Here's how the part is built. I have some questions about the finished solid (model axes, mm). A direction names the side the tool comes from. Round coordinates to 2 decimals unless told otherwise and drop trailing zeros. Order: outer loops, then holes, each group sorted by start corner. A loop starts at its lowest first (then second) coordinate and runs counter-clockwise, first axis right, second up. Notation, with made-up numbers: (62, 82) - (108, 82) arc R15 ccw to (108, 104) - close; hole circle Ø11 at (58, 71.25). An arc over 180 degrees is marked (long way). One line per item, written item: value.
from build123d import *

# Parameters (mm, degrees)
CROQUIS2_R                 = 1.6
SALIENTE_EXTRUIR1_DEPTH    = 15.1
CORTAR_EXTRUIR4_DEPTH      = 8.1
CORTAR_EXTRUIR2_DEPTH      = 37.049965326
CORTAR_EXTRUIR2_DEPTH_BACK = 4
CROQUIS4_R                 = 3.25
CORTAR_EXTRUIR3_DEPTH      = 4
REDONDEO2_R                = 1
CHAFL_N1_SIZE              = 0.5


with BuildPart() as part:
    # Croquis2 → Saliente-Extruir1 (new, symmetric)
    with BuildSketch(Plane(origin=(0, 0, 0), x_dir=(0, 0, -1), z_dir=(0, 1, 0))):
        with BuildLine():
            Line((0, -7), (0, 7))
            Line((0, 7), (-9, 7))
            Line((-9, 7), (-9, 5.817215829))
            ThreePointArc((-9, 5.817215829), (-9.710647783, 4.541706881), (-11.169230769, 4.474781407))
            ThreePointArc((-11.169230769, 4.474781407), (-18.4, 0), (-11.169230769, -4.474781407))
            ThreePointArc((-11.169230769, -4.474781407), (-9.710647783, -4.541706881), (-9, -5.817215829))
            Line((-9, -5.817215829), (-9, -7))
            Line((-9, -7), (0, -7))
        make_face()
        with Locations(Location((-13.4, 0, 0), (0, 0, 180))):
            Circle(CROQUIS2_R, mode=Mode.SUBTRACT)
    extrude(amount=SALIENTE_EXTRUIR1_DEPTH, both=True)

    # Croquis6 → Cortar-Extruir4 (cut, symmetric)
    with BuildSketch(Plane(origin=(0, 0, 0), x_dir=(1, 0, 0), z_dir=(0, 1, 0))):
        with BuildLine():
            Line((-7, -9), (-3.3, -9))
            ThreePointArc((-3.3, -9), (0, -7.9), (3.3, -9))
            Line((3.3, -9), (7, -9))
            Line((7, -9), (7, -18.9))
            Line((7, -18.9), (-7, -18.9))
            Line((-7, -18.9), (-7, -9))
        make_face()
    extrude(amount=CORTAR_EXTRUIR4_DEPTH, both=True, mode=Mode.SUBTRACT)

    # Croquis4 → Cortar-Extruir2 (cut, two sides: drawn at the far end of the back side and taken through both)
    with BuildSketch(Plane(origin=(0, 15.1, 0), x_dir=(1, 0, 0), z_dir=(0, 1, 0)).offset(-CORTAR_EXTRUIR2_DEPTH_BACK)):
        with Locations(Location((0, -13.4, 0), (0, 0, 90))):
            Circle(CROQUIS4_R)
    extrude(amount=CORTAR_EXTRUIR2_DEPTH + CORTAR_EXTRUIR2_DEPTH_BACK, mode=Mode.SUBTRACT)

    # Croquis5 → Cortar-Extruir3 (cut)
    with BuildSketch(Plane.XZ.offset(15.1)):
        Polygon((1.5011107, 10.8), (3.0022214, 13.4), (1.5011107, 16), (-1.5011107, 16), (-3.0022214, 13.4), (-1.5011107, 10.8), align=None)
    extrude(amount=-CORTAR_EXTRUIR3_DEPTH, mode=Mode.SUBTRACT)

    # Redondeo2
    redondeo2_edges = [part.edges().sort_by_distance(p)[0] for p in [
        (7, 0, 9),
        (-7, 0, 9),
    ]]
    fillet(redondeo2_edges, radius=REDONDEO2_R)

    # Chaflán1
    # the kernel refuses this chamfer: 0.5 mm, written as the material it takes off along each edge
    with BuildSketch(Plane(origin=(0, -15.1, 13.4), x_dir=(-0.8949562813691682, 0, -0.44615384615384657), z_dir=(0.44615384615384657, 0, -0.8949562813691682))) as chafl_n1_piece_1:
        Polygon((5 - CHAFL_N1_SIZE, 0), (5, CHAFL_N1_SIZE), (5, 0), align=None)
    revolve(axis=Axis((0, -15.1, 13.4), (0, 1, 0)), revolution_arc=232.994370335, mode=Mode.SUBTRACT)
    with BuildSketch(Plane(origin=(-5.817215829, -15.1, 10.5), x_dir=(0, 0, -1), z_dir=(-1, 0, 0))) as chafl_n1_piece_2:
        Polygon((1.5 + CHAFL_N1_SIZE, 0), (1.5, -CHAFL_N1_SIZE), (1.5, 0), align=None)
    revolve(axis=Axis((-5.817215829, -15.1, 10.5), (0, -1, 0)), revolution_arc=116.497185168, mode=Mode.SUBTRACT)
    with BuildSketch(Plane(origin=(-7, -15.1, -1.285841494), x_dir=(0.9996219169112968, -0.027495876610585647, 0), z_dir=(0, 0, 1)), Plane(origin=(-7, 15.1, -1.285841494), x_dir=(-0.027495876610585647, -0.9996219169112968, 0), z_dir=(0, 0, 1)), Plane(origin=(7, -15.1, 8), x_dir=(-0.9996219169112968, -0.027495876610585647, 0), z_dir=(0, 0, -1)), Plane(origin=(7, 15.1, 8), x_dir=(0.027495876610585647, -0.9996219169112968, 0), z_dir=(0, 0, -1))) as chafl_n1_piece_3:
        Polygon((CHAFL_N1_SIZE * 0.999621916911, CHAFL_N1_SIZE * 0.0274958766106), (-CHAFL_N1_SIZE * 0.0274958766106, CHAFL_N1_SIZE * 0.999621916911), (0, 0), align=None)
    extrude(amount=9.285841494, mode=Mode.SUBTRACT)
    with BuildSketch(Plane(origin=(-5.817215829, 15.1, 10.5), x_dir=(0, 0, -1), z_dir=(-1, 0, 0))) as chafl_n1_piece_4:
        Polygon((1.5 + CHAFL_N1_SIZE, 0), (1.5, CHAFL_N1_SIZE), (1.5, 0), align=None)
    revolve(axis=Axis((-5.817215829, 15.1, 10.5), (0, -1, 0)), revolution_arc=116.497185168, mode=Mode.SUBTRACT)
    with BuildSketch(Plane(origin=(0, 15.1, 13.4), x_dir=(-0.8949562813691682, 0, -0.44615384615384657), z_dir=(0.44615384615384657, 0, -0.8949562813691682))) as chafl_n1_piece_5:
        Polygon((5 - CHAFL_N1_SIZE, 0), (5, -CHAFL_N1_SIZE), (5, 0), align=None)
    revolve(axis=Axis((0, 15.1, 13.4), (0, 1, 0)), revolution_arc=232.994370335, mode=Mode.SUBTRACT)
    with BuildSketch(Plane(origin=(5.817215829, 15.1, 10.5), x_dir=(-0.8949562813691686, 0, 0.44615384615384585), z_dir=(0.44615384615384585, 0, 0.8949562813691686))) as chafl_n1_piece_6:
        Polygon((1.5 + CHAFL_N1_SIZE, 0), (1.5, CHAFL_N1_SIZE), (1.5, 0), align=None)
    revolve(axis=Axis((5.817215829, 15.1, 10.5), (0, -1, 0)), revolution_arc=116.497185168, mode=Mode.SUBTRACT)
    with BuildSketch(Plane(origin=(5.817215829, 15.1, 9), x_dir=(0, -0.9996219169112968, 0.027495876610585647), z_dir=(1, 0, 0)), Plane(origin=(-6, -15.1, 9), x_dir=(0, -0.027495876610585647, -0.9996219169112968), z_dir=(1, 0, 0)), Plane(origin=(-6, 15.1, 9), x_dir=(0, -0.9996219169112968, 0.027495876610585647), z_dir=(1, 0, 0)), Plane(origin=(5.817215829, -15.1, 9), x_dir=(0, -0.027495876610585647, -0.9996219169112968), z_dir=(1, 0, 0))) as chafl_n1_piece_7:
        Polygon((CHAFL_N1_SIZE * 0.999621916911, CHAFL_N1_SIZE * 0.0274958766106), (-CHAFL_N1_SIZE * 0.0274958766106, CHAFL_N1_SIZE * 0.999621916911), (0, 0), align=None)
    extrude(amount=0.182784171, mode=Mode.SUBTRACT)
    with BuildSketch(Plane(origin=(-5.817215829, 8.1, 10.5), x_dir=(0.8949562813691686, 0, 0.44615384615384585), z_dir=(-0.44615384615384585, 0, 0.8949562813691686))) as chafl_n1_piece_8_section:
        Polygon((1.5 + CHAFL_N1_SIZE, 0), (1.5, CHAFL_N1_SIZE), (1.5, 0), align=None)
    chafl_n1_piece_8 = revolve(axis=Axis((-5.817215829, 8.1, 10.5), (0, 1, 0)), revolution_arc=165.645776503, mode=Mode.PRIVATE)
    chafl_n1_piece_8 = split(chafl_n1_piece_8, bisect_by=Plane(origin=(-4.168851262, 8.241008039, 9), z_dir=(0, 0, 1)), keep=Keep.TOP, mode=Mode.PRIVATE)
    add(chafl_n1_piece_8, mode=Mode.SUBTRACT)
    with BuildSketch(Plane(origin=(0, 8.1, 13.4), x_dir=(-0.8949562813691682, 0, -0.44615384615384657), z_dir=(0.44615384615384657, 0, -0.8949562813691682))) as chafl_n1_piece_9:
        Polygon((5 - CHAFL_N1_SIZE, 0), (5, CHAFL_N1_SIZE), (5, 0), align=None)
    revolve(axis=Axis((0, 8.1, 13.4), (0, 1, 0)), revolution_arc=232.994370335, mode=Mode.SUBTRACT)
    with BuildSketch(Plane(origin=(5.817215829, 8.1, 10.5), x_dir=(0.7564084690774899, 0, -0.6540995550433039), z_dir=(0.6540995550433039, 0, 0.7564084690774899))) as chafl_n1_piece_10_section:
        Polygon((1.5, CHAFL_N1_SIZE), (1.5 + CHAFL_N1_SIZE, 0), (1.5, 0), align=None)
    chafl_n1_piece_10 = revolve(axis=Axis((5.817215829, 8.1, 10.5), (0, 1, 0)), revolution_arc=165.645776503, mode=Mode.PRIVATE)
    chafl_n1_piece_10 = split(chafl_n1_piece_10, bisect_by=Plane(origin=(4.495767194, 8.276282953, 9), z_dir=(0, 0, 1)), keep=Keep.TOP, mode=Mode.PRIVATE)
    add(chafl_n1_piece_10, mode=Mode.SUBTRACT)
    with BuildSketch(Plane(origin=(-5.817215829, -8.1, 10.5), x_dir=(0.8949562813691686, 0, 0.44615384615384585), z_dir=(-0.44615384615384585, 0, 0.8949562813691686))) as chafl_n1_piece_11_section:
        Polygon((1.5, -CHAFL_N1_SIZE), (1.5 + CHAFL_N1_SIZE, 0), (1.5, 0), align=None)
    chafl_n1_piece_11 = revolve(axis=Axis((-5.817215829, -8.1, 10.5), (0, 1, 0)), revolution_arc=165.645776503, mode=Mode.PRIVATE)
    chafl_n1_piece_11 = split(chafl_n1_piece_11, bisect_by=Plane(origin=(-4.495767364, -8.276282993, 9), z_dir=(0, 0, 1)), keep=Keep.TOP, mode=Mode.PRIVATE)
    add(chafl_n1_piece_11, mode=Mode.SUBTRACT)
    with BuildSketch(Plane(origin=(0, -8.1, 13.4), x_dir=(-0.8949562813691682, 0, -0.44615384615384657), z_dir=(0.44615384615384657, 0, -0.8949562813691682))) as chafl_n1_piece_12:
        Polygon((5, -CHAFL_N1_SIZE), (5 - CHAFL_N1_SIZE, 0), (5, 0), align=None)
    revolve(axis=Axis((0, -8.1, 13.4), (0, 1, 0)), revolution_arc=232.994370335, mode=Mode.SUBTRACT)
    with BuildSketch(Plane(origin=(5.817215829, -8.1, 10.5), x_dir=(0.7564084690774899, 0, -0.6540995550433039), z_dir=(0.6540995550433039, 0, 0.7564084690774899))) as chafl_n1_piece_13_section:
        Polygon((1.5, -CHAFL_N1_SIZE), (1.5 + CHAFL_N1_SIZE, 0), (1.5, 0), align=None)
    chafl_n1_piece_13 = revolve(axis=Axis((5.817215829, -8.1, 10.5), (0, 1, 0)), revolution_arc=165.645776503, mode=Mode.PRIVATE)
    chafl_n1_piece_13 = split(chafl_n1_piece_13, bisect_by=Plane(origin=(4.495767194, -8.276282953, 9), z_dir=(0, 0, 1)), keep=Keep.TOP, mode=Mode.PRIVATE)
    add(chafl_n1_piece_13, mode=Mode.SUBTRACT)
    with BuildSketch(Plane(origin=(6, -15.1, 8), x_dir=(1, 0, 0), z_dir=(0, 0, -1))) as chafl_n1_piece_14:
        Polygon((1 - CHAFL_N1_SIZE, 0), (1, -CHAFL_N1_SIZE), (1, 0), align=None)
    revolve(axis=Axis((6, -15.1, 8), (0, -1, 0)), revolution_arc=90, mode=Mode.SUBTRACT)
    with BuildSketch(Plane(origin=(-6, -15.1, 8), x_dir=(-1, 0, 0), z_dir=(0, 0, -1))) as chafl_n1_piece_15:
        Polygon((1 - CHAFL_N1_SIZE, 0), (1, CHAFL_N1_SIZE), (1, 0), align=None)
    revolve(axis=Axis((-6, -15.1, 8), (0, 1, 0)), revolution_arc=90, mode=Mode.SUBTRACT)
    with BuildSketch(Plane(origin=(6, 15.1, 8), x_dir=(1, 0, 0), z_dir=(0, 0, -1))) as chafl_n1_piece_16:
        Polygon((1, CHAFL_N1_SIZE), (1 - CHAFL_N1_SIZE, 0), (1, 0), align=None)
    revolve(axis=Axis((6, 15.1, 8), (0, -1, 0)), revolution_arc=90, mode=Mode.SUBTRACT)
    with BuildSketch(Plane(origin=(5.817215829, -15.1, 10.5), x_dir=(-0.8949562813691686, 0, 0.44615384615384585), z_dir=(0.44615384615384585, 0, 0.8949562813691686))) as chafl_n1_piece_17:
        Polygon((1.5 + CHAFL_N1_SIZE, 0), (1.5, -CHAFL_N1_SIZE), (1.5, 0), align=None)
    revolve(axis=Axis((5.817215829, -15.1, 10.5), (0, -1, 0)), revolution_arc=116.497185168, mode=Mode.SUBTRACT)
    with BuildSketch(Plane(origin=(-6, 15.1, 8), x_dir=(-1, 0, 0), z_dir=(0, 0, -1))) as chafl_n1_piece_18:
        Polygon((1, -CHAFL_N1_SIZE), (1 - CHAFL_N1_SIZE, 0), (1, 0), align=None)
    revolve(axis=Axis((-6, 15.1, 8), (0, 1, 0)), revolution_arc=90, mode=Mode.SUBTRACT)


solid = part.part
Q1. If we section it at C-C, the plane z = 13: Give the number of separate pieces and of enclosed holes in the cut face, then the cut area to 3 significant figures.
Results list:
separate pieces: 4
enclosed holes: 0
area: 72.0 mm²
Q2. If we section it at A-A, the plane x = 0: Please give me the cut outline in (y, z).
Results list:
outline: (-15.1, 0) - (15.1, 0) - (15.1, 10.15) - (11.1, 10.15) - (11.1, 11.8) - (8.1, 11.8) - (8.1, 7.9) - (-8.1, 7.9) - (-8.1, 11.8) - (-11.1, 11.8) - (-11.1, 10.8) - (-15.1, 10.8) - close; (-15.1, 16) - (-11.1, 16) - (-11.1, 15) - (-8.1, 15) - (-8.1, 17.9) - (-8.6, 18.4) - (-14.6, 18.4) - (-15.1, 17.9) - close; (8.1, 15) - (11.1, 15) - (11.1, 16.65) - (15.1, 16.65) - (15.1, 17.9) - (14.6, 18.4) - (8.6, 18.4) - (8.1, 17.9) - close
Q3. If we section it at B-B, the plane y = 10: Please give me the cut outline in (x, z), then the cut area to 3 significant figures.
Results list:
outline: (-7, 0) - (7, 0) - (7, 8) arc R1 ccw to (6, 9) - (5.82, 9) arc R1.5 cw to (4.47, 11.17) arc R5 ccw (long way) to (-4.47, 11.17) arc R1.5 cw to (-5.82, 9) - (-6, 9) arc R1 ccw to (-7, 8) - close; hole circle Ø3.2 at (0, 13.4)
area: 198 mm²
Q4. Will these pins go through, and if not, where does the flat tip stop? pin 1 (4 mm diameter, centred on x = 0, z = 13.4, fed in from -Y); pin 2 (2.5 mm diameter, centred on x = 0, z = 13.4, fed in from +Y); pin 3 (4 mm diameter, centred on x = -5.5, y = -3, fed in from +Z); pin 4 (3 mm diameter, centred on y = 11.5, z = 10, fed in from +X).
Results list:
pin 1: y = -11.1
pin 2: through
pin 3: z = 9
pin 4: x = 6.87
Q5. We'd pull the mould along Z, two halves only. Please class faces 4 (the flat face through (0, -15.1, 7)), 5 (the cylindrical face through (0, 10, 15)), 6 (the cylindrical face through (-4.553, 11.642, 9.693)), 7 (the flat face through (5, 0, 9)): released by +Z, released by -Z, zero draft, split by the parting line, or undercut.
Results list:
face 4: zero draft
face 5: undercut
face 6: undercut
face 7: released by +Z
Q6. If I drill on line 1 along Z through (x, y) = (0, -8.9); line 2 along Y through (x, z) = (2, 12.5); line 3 along X through (y, z) = (12.25, 13.4), over which ranges is the centre line in solid material (lowest first)?
Results list:
line 1: 0 to 11.8, 15 to 18.4
line 2: -11.1 to -8.1, 8.1 to 11.1
line 3: -5 to -3.25, 3.25 to 5
Q7. Which directions (+Z, -Z, +X, -X, +Y, -Y) give clear straight access to the entire face, cutting with the end or side of a thin tool? Please do faces 1 (the cylindrical face through (-0.1, 11.6, 18.4)), 2 (the flat face through (-2.262, -13.128, 12.118)), 3 (the flat face through (1, 11.1, 15)).
Results list:
face 1: +Y, -Y
face 2: -Y
face 3: +Y
